Autodesk Inventor part; units mm, degrees
ref_plane "YZ Plane" through (0, 0, 0) normal (1, 0, 0) x (0, 1, 0)
ref_plane "XZ Plane" through (0, 0, 0) normal (0, 1, 0) x (-1, 0, 0)
ref_plane "XY Plane" through (0, 0, 0) normal (0, 0, 1) x (1, 0, 0)
sketch "Skizze1" plane through (0, 0, 0) normal (0, 1, 0) x (-1, 0, 0)
  circle A0 centre (0, 0) radius 3
  line L0 (-20, -4) -> (20, -4)
  line L1 (20, -4) -> (20, 4)
  line L2 (20, 4) -> (-20, 4)
  line L3 (-20, 4) -> (-20, -4)
  line L4 (-20, -4) -> (20, 4) construction
  line L5 (20, -4) -> (-20, 4) construction
  dimension "d0" = 6
  dimension "d1" = 40
  dimension "d2" = 8
extrude "Extrusion1" add sketch "Skizze1" along normal blind 10
sketch "Skizze2" plane through (0, 0, 0) normal (0, 1, 0) x (-1, 0, 0)
  circle A0 centre (0, 0) radius 127
  circle A1 centre (0, 0) radius 3
  dimension "d6" = 254
extrude "Extrusion2" add sketch "Skizze2" along normal blind 10
chamfer "Fase1" distance 100 angle 5 1 edges at (127, 0, 0) measured on face at (84.8365, 0, -10.6241)
equation "\"G_L\" = 0"
equation "\"G_H\" = 0"
equation "\"G_B\" = 0"
properties part number "Props" material "GEDA Plexiglas"
Can you work these out from the model? Positions are in its coordinate system, mm. Coordinates: 2 decimals unless noted, no trailing zeros. Loops run counter-clockwise (first coordinate to the right, second up) from the corner with the lowest first, then second, coordinate; pieces in that order, holes last.
1) I need wall thicknesses on probe 1 along Y at (x, z) = (-39, 82); probe 2 along Y at (x, z) = (-97, 5); probe 3 along Z at (x, y) = (51, 9.75). Which ranges of each line are inside material? Lowest first, please.
2) Imagine slicing it at A-A on x = 0. List the corners of the cut face in (y, z) for me, plus the area to 3 significant figures.
3) Thinking about a two-plate mould opening in Z: for faces 1 (the cylindrical face through (3, 5, 0)), 2 (the flat face through (-6, 0, 0)), 3 (the conical face through (7.209, 0.547, -32.465)), which applies, pulls with the +Z half, pulls with the -Z half, needs draft (parallel to the pull), parting line crosses it, or undercut?
4) For pin 1 (8 mm diameter, centred on x = 0, z = 0, fed in from -Y); pin 2 (6 mm diameter, centred on x = 55, z = -29.5, fed in from -Y), each with a flat end and sliding along its axis, tell me the tip position at first contact or that it passes through.
5) Imagine slicing it at C-C on y = 6.5. List the corners of the cut face in (x, z) for me.
6) Imagine slicing it at B-B on z = 0. List the corners of the cut face in (x, y) for me, plus the area to 3 significant figures.
Completed:
1. probe 1: y = 5.58 to 10
1. probe 2: y = 6.14 to 10
1. probe 3: z = -116.31 to 116.31
2. outline: (0, -27) - (8.75, -127) - (10, -127) - (10, -3) - (0, -3) - close; (0, 3) - (10, 3) - (10, 127) - (8.75, 127) - (0, 27) - close
2. area: 1,610 mm2
3. face 1: undercut
3. face 2: needs draft
3. face 3: parting line crosses it
4. pin 1: stops at y = 0
4. pin 2: stops at y = 2.84
5. outline: circle Ø202.59 at (0, 0); hole circle Ø6 at (0, 0)
6. outline: (-127, 8.75) - (-27, 0) - (-3, 0) - (-3, 10) - (-127, 10) - close; (3, 0) - (27, 0) - (127, 8.75) - (127, 10) - (3, 10) - close
6. area: 1,610 mm2
